Model file for the job. Use its own axes, mm. Face numbers are marked on the shaded views. A direction names the side the tool comes from. Round coordinates to 2 decimals unless told otherwise and drop trailing zeros. Order: outer loops, then holes, each group sorted by start corner. A loop starts at its lowest first (then second) coordinate and runs counter-clockwise, first axis right, second up. Notation, with made-up numbers: (58, -21) - (107, -21) arc R11 cw to (107, -10) - close; hole circle Ø5 at (10, -29.5). An arc over 180 degrees is marked (long way). Write item = value, one per line.
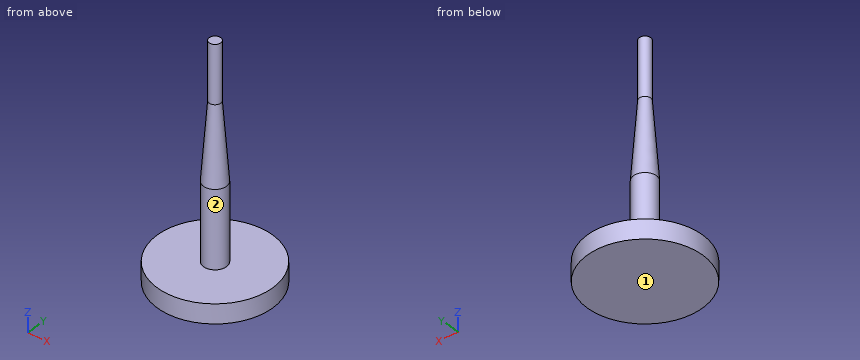
```python
from build123d import *

# Parameters (mm, degrees)
F0_R     = 38.1
F1_DEPTH = 12.7
F2_R     = 7.62
F3_DEPTH = 50.8
F6_DEPTH = 38.1


# Not quite as in the source:
# - a feature names something its author has since deleted; it is built from what else it names


with BuildPart() as f1:
    # F0 (on Top) → F1 (new body)
    with BuildSketch(Plane.XY):
        Circle(F0_R)
    extrude(amount=F1_DEPTH)

    # F2 (on face) → F3 (join)
    with BuildSketch(Plane.XY.offset(12.7)):
        Circle(F2_R)
    extrude(amount=F3_DEPTH)

    # F4 (on Right) → F5 (revolve)
    with BuildSketch(Plane.YZ):
        Polygon((0, 114.3), (0, 63.5), (7.62, 63.5), (3.81, 114.3), align=None)
    revolve(axis=Axis((0, 0, 88.9), (0, 0, 1)))

    # F6 (add): a face of the model
    f6_faces = [f1.faces().sort_by_distance(p)[0] for p in [
        (0, 0, 114.3),
    ]]
    extrude(f6_faces, amount=F6_DEPTH)


solid = f1.part
```
1) Cut at A-A (y = 0). Write the cut outline in (x, z).
Conclusion:
outline = (-38.1, 0) - (38.1, 0) - (38.1, 12.7) - (7.62, 12.7) - (7.62, 63.5) - (3.81, 114.3) - (3.81, 152.4) - (-3.81, 152.4) - (-3.81, 114.3) - (-7.62, 63.5) - (-7.62, 12.7) - (-38.1, 12.7) - close
2) Wall check: line 1 along Z through (x, y) = (2.5, 8); line 2 along X through (y, z) = (0.5, 138); line 3 along Y through (x, z) = (2, 58). Give the ranges that are in metal, low to high.
Conclusion:
line_1 = 0 to 12.7
line_2 = -3.78 to 3.78
line_3 = -7.35 to 7.35
3) Flat gauge pins, fed straight in: pin 1 Ø6 at (y, z) = (18.5, 18.5) entering from -X (3 decimals); pin 2 Ø10 at (x, y) = (-25, 26.5) entering from +Z; pin 3 Ø3 at (y, z) = (5, 59) entering from +X; pin 4 Ø1.5 at (x, z) = (-3.5, 100) entering from -Y. Where does each tip first touch, or does it go through?
Conclusion:
pin_1 = through
pin_2 = 12.7
pin_3 = 6.77
pin_4 = -4.04
4) Cut at C-C (z = 131). Write the cut outline in (x, y), and give its area (3 significant figures).
Conclusion:
outline = circle Ø7.62 at (0, 0)
area = 45.6 mm^2
5) Cut at D-D (z = 51). Write the cut outline in (x, y), and give its area (3 significant figures).
Conclusion:
outline = circle Ø15.24 at (0, 0)
area = 182 mm^2
6) 3-axis set-ups, long thin cutter, end or side, ignore diameter. For the marked faces 1 and 2: which of +Z, -Z, +X, -X, +Y, -Y reach the whole face in a straight line?
Conclusion:
face_1 = -Z, +X, -X, +Y, -Y
face_2 = +Z
